Check sheet for the modelled part. Datum: model origin and axes. Units: mm. Face numbers are marked on the shaded views. A direction names the side the tool comes from. Coordinates: 2 decimals unless noted, no trailing zeros. Order: outer loops, then holes, each group sorted by start corner. A loop starts at its lowest first (then second) coordinate and runs counter-clockwise, first axis right, second up.
1. Cross-section at A-A (z = 0). Count the separate pieces of the cut face and the enclosed holes in it, then the cut area to 3 significant figures.
2. Thickness scan on line 1 (X direction, y = 7.6, z = 0); line 2 (X direction, y = 5.75, z = -4); line 3 (Y direction, x = 17, z = 0.5). Record the ranges inside material, lowest first.
3. Cross-section at C-C (x = -2). Enter the section's corners in (y, z).
4. Gauge pin test, flat ends, axial feed: pin 1 Ø6 at (x, z) = (17, 1) entering from +Y; pin 2 Ø1 at (x, y) = (11, -6.5) entering from +Z; pin 3 Ø8 at (x, z) = (5.5, 3) entering from +Y; pin 4 Ø0.6 at (y, z) = (7.5, 1) entering from -X. Record the tip position at first contact, or that the pin passes through.
5. Draft check along X on the marked faces 6, 7 and 8. Enter one of: released by +X, released by -X, zero draft, split by the parting line, or undercut.
6. Cross-section at B-B (y = -3.5). Enter the section's corners in (x, z).
7. Set-up check for the marked faces 1, 2, 3, 4 and 5: record each of +Z, -Z, +X, -X, +Y, -Y from which the full face is reachable in a straight line by a thin tool's end or side.
```python
from build123d import *

# Parameters (mm, degrees)
SKETCH1_W       = 22.352
SKETCH1_H       = 7.874
EXTRUDE1_DEPTH  = 6.985
EXTRUDE2_DEPTH  = 0.5588
SKETCH3_W       = 11.811
SKETCH3_H       = 6.096
EXTRUDE3_DEPTH  = 0.762
SKETCH4_W       = 7.0612
SKETCH4_H       = 5.6896
EXTRUDE4_DEPTH  = 9.4996
SKETCH7_W       = 7.9248
SKETCH7_H       = 5.6896
EXTRUDE7_DEPTH  = 0.762
FILLET2_R       = 1.27
SKETCH5_R       = 1.778
EXTRUDE5_DEPTH  = 9.4996
SKETCH6_R       = 0.9144
EXTRUDE6_DEPTH  = 0.508
LPATTERN1_COUNT = 2
LPATTERN1_PITCH = 7.9248
LPATTERN2_COUNT = 2
LPATTERN2_PITCH = 7.9248


with BuildPart() as part:
    # Sketch1 → Extrude1 (new, symmetric)
    with BuildSketch(Plane.XY):
        with Locations((11.176, 3.937)):
            Rectangle(SKETCH1_W, SKETCH1_H)
    extrude(amount=EXTRUDE1_DEPTH, both=True)

    # Sketch2 → Extrude2 (add)
    with BuildSketch(Plane(origin=(0, 7.874, 0), x_dir=(1, 0, 0), z_dir=(0, 1, 0))):
        with BuildLine():
            Line((0, 6.35), (-5.3848, 3.24108427))
            ThreePointArc((-5.3848, 3.24108427), (-6.096, 0), (-5.3848, -3.24108427))
            Line((-5.3848, -3.24108427), (0, -6.35))
            Line((0, -6.35), (0, 6.35))
        make_face()
        with BuildLine():
            Line((22.352, 6.35), (22.352, -6.35))
            Line((22.352, -6.35), (27.7368, -3.24108427))
            ThreePointArc((27.7368, -3.24108427), (28.448, 0), (27.7368, 3.24108427))
            Line((27.7368, 3.24108427), (22.352, 6.35))
        make_face()
    extrude(amount=-EXTRUDE2_DEPTH)

    # Sketch3 → Extrude3 (cut)
    with BuildSketch(Plane(origin=(0, 7.874, 0), x_dir=(1, 0, 0), z_dir=(0, 1, 0))):
        with Locations((11.176, 0)):
            Rectangle(SKETCH3_W, SKETCH3_H)
    extrude(amount=-EXTRUDE3_DEPTH, mode=Mode.SUBTRACT)

    # Sketch4 → Extrude4 (add)
    with BuildSketch(Plane(origin=(0, 7.112, 0), x_dir=(1, 0, 0), z_dir=(0, 1, 0))):
        with Locations((12.8143, 0)):
            Rectangle(SKETCH4_W, SKETCH4_H)
    extrude(amount=EXTRUDE4_DEPTH)

    # Sketch7 → Extrude7 (add)
    with BuildSketch(Plane(origin=(0, 7.874, 0), x_dir=(1, 0, 0), z_dir=(0, 1, 0))):
        with Locations((12.8143, 0)):
            Rectangle(SKETCH7_W, SKETCH7_H)
    extrude(amount=-EXTRUDE7_DEPTH)

    # Fillet2
    fillet2_edges = [part.edges().sort_by_distance(p)[0] for p in [
        (9.2837, 16.6116, 0),
        (16.3449, 16.6116, 0),
    ]]
    fillet(fillet2_edges, radius=FILLET2_R)

    # Sketch5 → Extrude5 (cut)
    with BuildSketch(Plane(origin=(0, 7.874, 0), x_dir=(1, 0, 0), z_dir=(0, 1, 0))):
        with Locations(Location((-3.1115, 0, 0), (0, 0, 270))):
            Circle(SKETCH5_R)
        with Locations(Location((25.4635, 0, 0), (0, 0, 270))):
            Circle(SKETCH5_R)
    extrude(amount=-EXTRUDE5_DEPTH, mode=Mode.SUBTRACT)

    # Sketch6 → Extrude6 (add)
    with BuildSketch(Plane.XY.offset(-1.27)):
        with BuildLine():
            Line((12.7635, -6.00209581), (12.7635, -8.548254179))
            ThreePointArc((12.7635, -8.548254179), (11.176, -9.144), (9.5885, -8.548254179))
            Line((9.5885, -8.548254179), (9.5885, 0))
            Line((9.5885, 0), (12.7635, 0))
            Line((12.7635, 0), (12.7635, -1.10990419))
            ThreePointArc((12.7635, -1.10990419), (11.533993687, -3.556), (12.7635, -6.00209581))
        make_face()
        with Locations((11.176, -7.493)):
            Circle(SKETCH6_R, mode=Mode.SUBTRACT)
    extrude6 = extrude(amount=-EXTRUDE6_DEPTH)

    # LPattern1: Extrude6 ×2
    with Locations(*[(i * LPATTERN1_PITCH, 0, 0) for i in range(1, LPATTERN1_COUNT)]):
        add(extrude6)

    # LPattern2: Extrude6 ×2
    with Locations(*[(-i * LPATTERN2_PITCH, 0, 0) for i in range(1, LPATTERN2_COUNT)]):
        add(extrude6)


solid = part.part
```
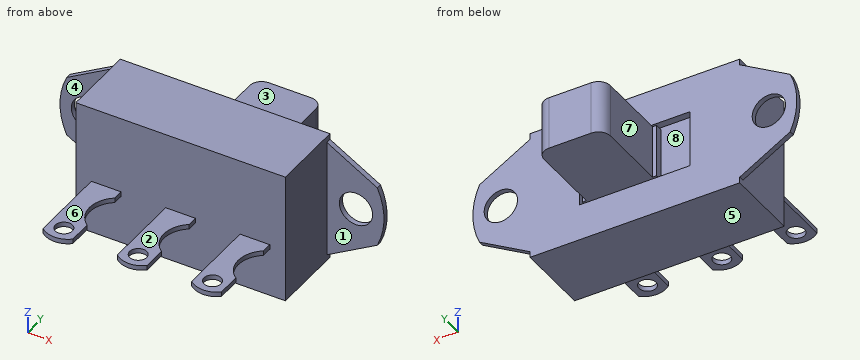
Data:
1. separate pieces: 3
1. enclosed holes: 0
1. area: 237 mm2
2. line 1: x = -6.1 to -4.89, -1.33 to 5.27, 8.85 to 16.78, 17.08 to 23.69, 27.24 to 28.45
2. line 2: x = 0 to 22.35
2. line 3: y = 0 to 7.11
3. outline: (7.32, -5.2) - (7.87, -5.2) - (7.87, -1.39) - (7.32, -1.39) - close; (7.32, 1.39) - (7.87, 1.39) - (7.87, 5.2) - (7.32, 5.2) - close
4. pin 1: stops at y = 16.61
4. pin 2: stops at z = -1.27
4. pin 3: stops at y = 16.05
4. pin 4: stops at x = -6.06
5. face 6: zero draft
5. face 7: released by -X
5. face 8: undercut
6. outline: (1.66, -1.78) - (3.61, -1.78) - (3.61, -1.27) - (1.66, -1.27) - close; (9.59, -1.78) - (11.53, -1.78) - (11.53, -1.27) - (9.59, -1.27) - close; (17.51, -1.78) - (19.46, -1.78) - (19.46, -1.27) - (17.51, -1.27) - close
7. face 1: +Z, -Z, +X, -Y
7. face 2: +Z, +X, -X, -Y
7. face 3: +Y
7. face 4: +Z, -Z, -X, -Y
7. face 5: -Z, +X, -X, +Y, -Y
